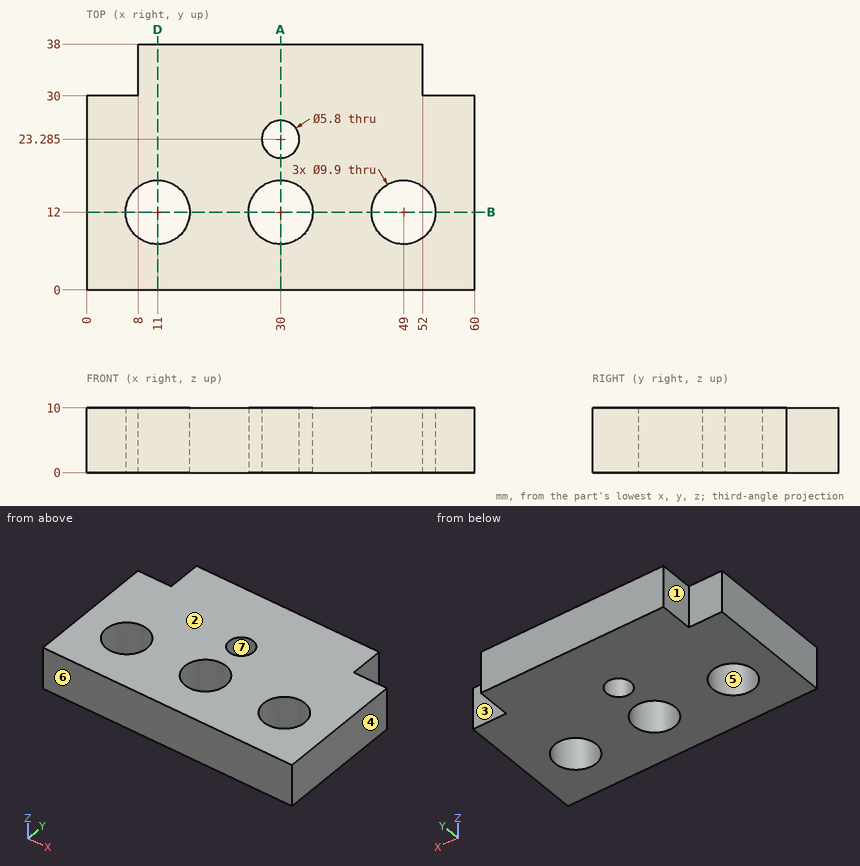
Geometry check sheet. Reference: drawing and pictorial views, mm from the part's lowest x, y, z. A direction names the side the tool comes from. Coordinates: 2 decimals unless noted, no trailing zeros. Loops run counter-clockwise (first coordinate to the right, second up) from the corner with the lowest first, then second, coordinate; pieces in that order, holes last. Notation, with made-up numbers: (-38, 21) -> (-14, 21) arc R13 cw to (-14, 28) -> close; hole circle Ø5 at (46, -30.75). An arc over 180 degrees is marked (long way). Put each result on its own line as item: value.
1) Gauge pin test, flat ends, axial feed: pin 1 Ø13 at (x, y) = (11, 12) entering from -Z; pin 2 Ø2.5 at (y, z) = (35.5, 3) entering from -X; pin 3 Ø2.5 at (y, z) = (32.5, 6.5) entering from +X; pin 4 Ø4 at (x, z) = (4, 4) entering from +Y. Record the tip position at first contact, or that the pin passes through.
Result set:
pin 1: stops at z = 0
pin 2: stops at x = 8
pin 3: stops at x = 52
pin 4: stops at y = 30
2) Cross-section at D-D on x = 11. Record the boundary of the cut face in (y, z), plus the area to 3 significant figures.
Result set:
outline: (0, 0) -> (7.05, 0) -> (7.05, 10) -> (0, 10) -> close; (16.95, 0) -> (38, 0) -> (38, 10) -> (16.95, 10) -> close
area: 281 mm^2
3) Cross-section at A-A on x = 30. Count the separate pieces of the cut face and the enclosed holes in it, plus the area to 3 significant figures.
Result set:
separate pieces: 3
enclosed holes: 0
area: 223 mm^2
4) Thickness scan on line 1 (X direction, y = 12, z = 2); line 2 (Y direction, x = 49, z = 5.75); line 3 (Y direction, x = 30.5, z = 8.5) (1 decimal). Record the ranges inside material, lowest first.
Result set:
line 1: x = 0 to 6.05, 15.95 to 25.05, 34.95 to 44.05, 53.95 to 60
line 2: y = 0 to 7.05, 16.95 to 38
line 3: y = 0 to 7.1, 16.9 to 20.4, 26.1 to 38
5) Tool access check on the marked faces 1, 2 and 3. Record the directions out of +Z, -Z, +X, -X, +Y, -Y that give a thin tool (end or side, any length) a straight path to the whole face; none if there is none.
Result set:
face 1: +Z, -Z, -X, +Y
face 2: +Z, +X, -X, +Y, -Y
face 3: +Z, -Z, +X, +Y
6) Cross-section at B-B on y = 12. Record the boundary of the cut face in (x, z).
Result set:
outline: (0, 0) -> (6.05, 0) -> (6.05, 10) -> (0, 10) -> close; (15.95, 0) -> (25.05, 0) -> (25.05, 10) -> (15.95, 10) -> close; (34.95, 0) -> (44.05, 0) -> (44.05, 10) -> (34.95, 10) -> close; (53.95, 0) -> (60, 0) -> (60, 10) -> (53.95, 10) -> close
7) Release check for a two-part mould opening along X. For the marked faces 4, 5, 6 and 7 record: released by +X, released by -X, zero draft, split by the parting line, or undercut.
Result set:
face 4: released by +X
face 5: undercut
face 6: zero draft
face 7: undercut
